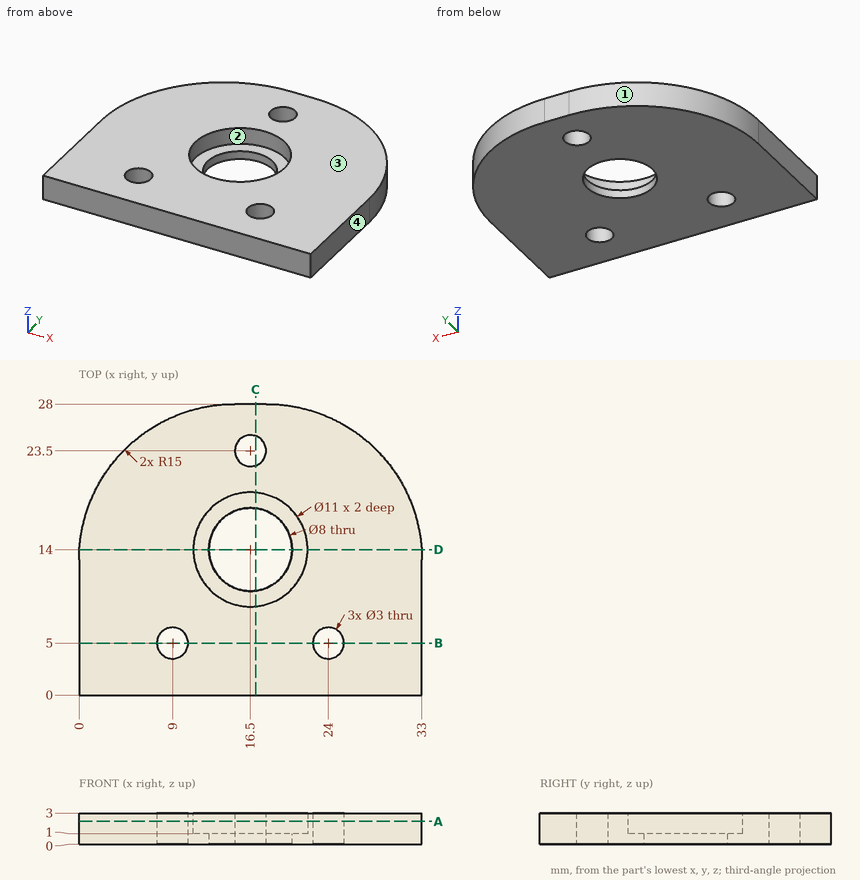
Part print with two shaded views. Sizes in mm from the minimum x, y, z corner. Round coordinates to 2 decimals unless told otherwise and drop trailing zeros. Write each loop counter-clockwise with the first axis right and the second up, starting at its lowest first coordinate (ties: lowest second). Pieces come first, ordered by that corner, then holes. Notation, with made-up numbers: (50, 17.5) -> (58, 17.5) arc R9 ccw to (58, 27.5) -> close; hole circle Ø1 at (38, -0.5). An arc over 180 degrees is marked (long way). Put each result on its own line as item: value.
Item 1: Two-plate mould, pull along X, no slides. Class the marked faces 1, 2, 3 and 4: pulls with the +X half, pulls with the -X half, needs draft (parallel to the pull), parting line crosses it, or undercut.
Here are the results:
face 1: pulls with the -X half
face 2: undercut
face 3: needs draft
face 4: pulls with the +X half
Item 2: Slice it at C-C, the plane x = 17. Give the cut face in (y, z).
Here are the results:
outline: (0, 0) -> (10.03, 0) -> (10.03, 1) -> (8.52, 1) -> (8.52, 3) -> (0, 3) -> close; (17.97, 0) -> (22.09, 0) -> (22.09, 3) -> (19.48, 3) -> (19.48, 1) -> (17.97, 1) -> close; (24.91, 0) -> (28, 0) -> (28, 3) -> (24.91, 3) -> close
Item 3: Wall check: probe 1 along Y at (x, z) = (16.5, 1.95); probe 2 along Y at (x, z) = (17, 1.6); probe 3 along Y at (x, z) = (24, 1.05). Give the ranges that are in metal, low to high. Write a range as from..to.
Here are the results:
probe 1: y = 0..8.5, 19.5..22, 25..28
probe 2: y = 0..8.52, 19.48..22.09, 24.91..28
probe 3: y = 0..3.5, 6.5..26.75
Item 4: Flat gauge pin, fed straight in: P1, Ø1.5, axis at x = 13, z = 1.5, coming from the +Y side. Where does the tip first touch, or does it go through?
Here are the results:
P1: stops at y = 27.95
Item 5: Slice it at B-B, the plane y = 5. Give the cut face in (x, z).
Here are the results:
outline: (0, 0) -> (7.5, 0) -> (7.5, 3) -> (0, 3) -> close; (10.5, 0) -> (22.5, 0) -> (22.5, 3) -> (10.5, 3) -> close; (25.5, 0) -> (33, 0) -> (33, 3) -> (25.5, 3) -> close
Item 6: Slice it at A-A, the plane z = 2.2. Give the cut face in (x, y), plus the area to 3 significant figures.
Here are the results:
outline: (0, 0) -> (33, 0) -> (33, 13) arc R15 ccw to (18, 28) -> (15, 28) arc R15 ccw to (0, 13) -> close; hole circle Ø3 at (9, 5); hole circle Ø11 at (16.5, 14); hole circle Ø3 at (16.5, 23.5); hole circle Ø3 at (24, 5)
area: 711 mm^2
Item 7: Slice it at D-D, the plane y = 14. Give the cut face in (x, z), plus the area to 3 significant figures.
Here are the results:
outline: (0.03, 0) -> (12.5, 0) -> (12.5, 1) -> (11, 1) -> (11, 3) -> (0.03, 3) -> close; (20.5, 0) -> (32.97, 0) -> (32.97, 3) -> (22, 3) -> (22, 1) -> (20.5, 1) -> close
area: 68.8 mm^2
